Geometry check sheet. Reference: drawing and pictorial views, mm from the part's lowest x, y, z. Coordinates: 2 decimals unless noted, no trailing zeros. Write each loop counter-clockwise with the first axis right and the second up, starting at its lowest first coordinate (ties: lowest second). Pieces come first, ordered by that corner, then holes. Notation, with made-up numbers: (37, 60.5) -> (44, 60.5) arc R14 cw to (44, 66.5) -> close; hole circle Ø6 at (44.5, -27.75). An arc over 180 degrees is marked (long way). Answer in a Markdown table with one row per item.
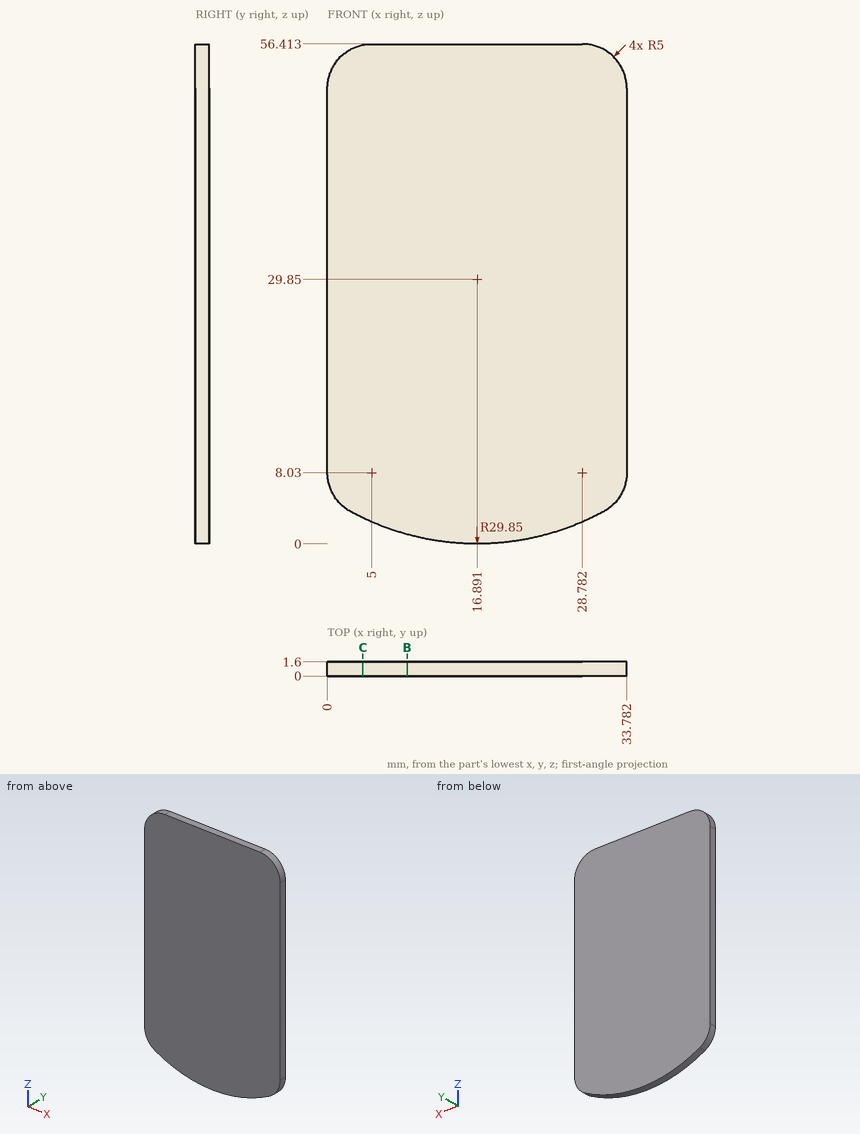
1. Section check B-B, the plane x = 9. Record the boundary of the cut face in (y, z).
Geometry says:
| item | result |
|---|---|
| outline | (0, 1.06) -> (1.6, 1.06) -> (1.6, 56.41) -> (0, 56.41) -> close |
2. Section check C-C, the plane x = 4. Record the boundary of the cut face in (y, z).
Geometry says:
| item | result |
|---|---|
| outline | (0, 2.93) -> (1.6, 2.93) -> (1.6, 56.31) -> (0, 56.31) -> close |
3. Thickness scan on line 1 (X direction, y = 1.5, z = 51.5); line 2 (Z direction, x = 8, y = 0.9) (1 decimal); line 3 (Z direction, x = 11, y = 1.05). Record the ranges inside material, lowest first. Write a range as from..to.
Geometry says:
| item | result |
|---|---|
| line 1 | 0..33.78 |
| line 2 | 1.4..56.4 |
| line 3 | 0.59..56.41 |
